Input: part model. Units: mm. Frame: model coordinates. A direction names the side the tool comes from. Coordinates: 2 decimals unless noted, no trailing zeros. Loops run counter-clockwise (first coordinate to the right, second up) from the corner with the lowest first, then second, coordinate; pieces in that order, holes last.
Item 1: Section C-C on x = 44.45. Return loops of the section in (y, z).
Item 2: Pull-direction query (Z, two-part tool) for faces 4 (the flat face through (0, 87.7, 99.5)), 5 (the flat face through (29, 83, 101.6)), 6 (the flat face through (20.29, 13.07, 93.31)), 7 (the flat face through (34, 168.91, 50)); classes: released by +Z, released by -Z, zero draft, split by the parting line, or undercut.
Item 3: Ray query, line 1 along Z through (x, y) = (6.5, 139.5); line 2 along Y through (x, z) = (11, 59.5); line 3 along X through (y, z) = (25, 100). Return the intervals inside material, ascending.
Item 4: Contact query for flat-ended pins moving along their axis: P1, Ø3, axis at y = 120.5, z = 100.5, coming from the -X side; P2, Ø3, axis at x = 47, z = 100.5, coming from the -Y side; P3, Ø1, axis at x = 50.5, z = 64, coming from the -Y side; P4, Ø20.5, axis at x = 31, z = 58, coming from the +Y side. Output: stop coordinate, or through.
Item 5: Section B-B on y = 25.4. Return loops of the section in (x, z).
Item 6: Reachability of faces 1 (the cylindrical face through (40.765, 28.779, 100.348)), 2 (the flat face through (16.51, 181, 50)), 3 (the flat face through (20.855, 161.783, 93.284)) from +Z, -Z, +X, -X, +Y, -Y: full face, straight path, thin tool, end or side. Return the list, or none.
Item 7: Section D-D on y = 132.5. Return loops of the section in (x, z), and give its area (3 significant figures).
Item 8: Section A-A on z = 68. Return loops of the section in (x, y), and give its area (3 significant figures).
```python
from build123d import *

# Parameters (mm, degrees)
BOSS_EXTRUDE2_DEPTH = 101.6
CUT_EXTRUDE1_DEPTH  = 58.15
SHELL1_T            = -2.54
SKETCH3_W           = 8.2
SKETCH3_H           = 4.8
SKETCH3_W_2         = 12
SKETCH3_H_2         = 5.75
CUT_EXTRUDE2_DEPTH  = 17.51
SKETCH4_W           = 5.75
SKETCH4_H           = 10
CUT_EXTRUDE3_DEPTH  = 27.94
SKETCH5_W           = 5.75
SKETCH5_H           = 12.75
CUT_EXTRUDE4_DEPTH  = 27.94
SKETCH6_R           = 5
CUT_EXTRUDE5_DEPTH  = 27.94


with BuildPart() as part:
    # Sketch1 → Boss-Extrude2 (new body)
    with BuildSketch(Plane.XY):
        Polygon((0, 0), (0, 190.5), (16.51, 190.5), (16.51, 171.45), (57.15, 171.45), (57.15, 19.05), (16.51, 0), align=None)
    extrude(amount=BOSS_EXTRUDE2_DEPTH)

    # Sketch2 → Cut-Extrude1 (cut, through all)
    with BuildSketch(Plane.ZY):
        Polygon((15.875, 190.5), (0, 146.05), (0, 190.5), align=None)
        Polygon((0, 19.05), (15.875, 0), (0, 0), align=None)
        Polygon((85.725, 0), (101.6, 19.05), (101.6, 0), align=None)
        Polygon((101.6, 146.05), (85.725, 190.5), (101.6, 190.5), align=None)
    extrude(amount=-CUT_EXTRUDE1_DEPTH, mode=Mode.SUBTRACT)

    # Shell1
    shell1_openings = [part.faces().sort_by_distance(p)[0] for p in [
        (0, 88.9, 50.8),
    ]]
    offset(amount=SHELL1_T, openings=shell1_openings, kind=Kind.INTERSECTION)

    # Sketch3 → Cut-Extrude2 (cut, through all)
    with BuildSketch(Plane(origin=(16.51, 0, 0), x_dir=(0, 0, -1), z_dir=(1, 0, 0))):
        with Locations((-70.147400598, 183.02)):
            Rectangle(SKETCH3_W, SKETCH3_H)
        with Locations((-29.56, 182.545)):
            Rectangle(SKETCH3_W_2, SKETCH3_H_2)
    extrude(amount=-CUT_EXTRUDE2_DEPTH, mode=Mode.SUBTRACT)

    # Sketch4 → Cut-Extrude3 (cut)
    with BuildSketch(Plane.XY.offset(101.6)):
        with Locations((45.385, 122)):
            Rectangle(SKETCH4_W, SKETCH4_H)
    extrude(amount=-CUT_EXTRUDE3_DEPTH, mode=Mode.SUBTRACT)

    # Sketch5 → Cut-Extrude4 (cut)
    with BuildSketch(Plane(origin=(0, 0, 0), x_dir=(-1, 0, 0), z_dir=(0, 0, -1))):
        with Locations((-45.385, 120.625)):
            Rectangle(SKETCH5_W, SKETCH5_H)
    extrude(amount=-CUT_EXTRUDE4_DEPTH, mode=Mode.SUBTRACT)

    # Sketch6 → Cut-Extrude5 (cut)
    with BuildSketch(Plane.XY.offset(101.6)):
        with Locations((44.45, 25.4)):
            Circle(SKETCH6_R)
    extrude(amount=-CUT_EXTRUDE5_DEPTH, mode=Mode.SUBTRACT)


solid = part.part
```
Results found:
1. outline: (13.1, 4.96) - (19.05, 0) - (114.25, 0) - (114.25, 2.54) - (19.97, 2.54) - (15.9, 5.93) - (15.9, 95.67) - (19.97, 99.06) - (20.4, 99.06) - (20.4, 101.6) - (19.05, 101.6) - (13.1, 96.64) - close; (30.4, 99.06) - (117, 99.06) - (117, 101.6) - (30.4, 101.6) - close; (127, 0) - (146.05, 0) - (171.45, 9.07) - (171.45, 92.53) - (146.05, 101.6) - (127, 101.6) - (127, 99.06) - (145.61, 99.06) - (168.91, 90.74) - (168.91, 10.86) - (145.61, 2.54) - (127, 2.54) - close
2. face 4: zero draft
2. face 5: released by +Z
2. face 6: undercut
2. face 7: undercut
3. line 1: z = 0 to 2.54, 99.06 to 101.6
3. line 2: y = 0 to 2.54, 187.96 to 190.5
3. line 3: x = 0 to 39.47, 49.43 to 57.15
4. P1: stops at x = 0
4. P2: stops at y = 15.93
4. P3: stops at y = 15.7
4. P4: stops at y = 171.45
5. outline: (0, 0) - (57.15, 0) - (57.15, 101.6) - (49.45, 101.6) - (49.45, 99.06) - (54.61, 99.06) - (54.61, 2.54) - (0, 2.54) - close; (0, 99.06) - (39.45, 99.06) - (39.45, 101.6) - (0, 101.6) - close
6. face 1: +Z
6. face 2: +Z, -Z, +X, +Y
6. face 3: -X
7. outline: (0, 0) - (57.15, 0) - (57.15, 101.6) - (0, 101.6) - (0, 99.06) - (54.61, 99.06) - (54.61, 2.54) - (0, 2.54) - close
7. area: 535 mm2
8. outline: (0, 0) - (16.51, 0) - (57.15, 19.05) - (57.15, 171.45) - (16.51, 171.45) - (16.51, 180.62) - (13.97, 180.62) - (13.97, 168.91) - (54.61, 168.91) - (54.61, 20.66) - (15.94, 2.54) - (0, 2.54) - close; (0, 187.96) - (13.97, 187.96) - (13.97, 185.42) - (16.51, 185.42) - (16.51, 190.5) - (0, 190.5) - close
8. area: 712 mm2
